Check sheet for the modelled part. Datum: model origin and axes. Units: mm. A direction names the side the tool comes from. Give positions to 0.01 mm unless a question says otherwise; leave off trailing zeros. Write each loop counter-clockwise with the first axis right and the second up, starting at its lowest first coordinate (ties: lowest second). Pieces come first, ordered by that corner, then holes. Notation, with made-up numbers: (26.5, 50) -> (73.5, 50) arc R31 ccw to (73.5, 81) -> close; hole circle Ø4 at (47.5, 87). An arc over 180 degrees is marked (long way). Use a Markdown table: item, result. Add a question column.
1. Set-up check for faces 4 (the flat face through (1.28, 21.51, 2.26)), 5 (the cylindrical face through (-3.417, 21.372, -0.759)): record each of +Z, -Z, +X, -X, +Y, -Y from which the full face is reachable in a straight line by a thin tool's end or side.
2. Release check for a two-part mould opening along Z. For faces 1 (the cylindrical face through (0.676, 9.86, 2.146)), 2 (the flat face through (3, 22, -1)), 3 (the flat face through (0, 21.016, 0)) record: released by +Z, released by -Z, zero draft, split by the parting line, or undercut.
3. Cross-section at B-B (y = 15.75). Enter the section's corners in (x, z), then the cut area to 3 significant figures.
4. Gauge pin test, flat ends, axial feed: P1, Ø1.5, axis at x = 0, y = 17, coming from the -Z side; P2, Ø1.6, axis at x = -1, z = 1, coming from the +Y side; P3, Ø2, axis at y = 3, z = 1, coming from the +X side. Record the tip position at first contact, or that the pin passes through.
5. Cross-section at A-A (z = 0). Enter the section's corners in (x, y), then the cut area to 3 significant figures.
6. Scan lines: probe 1 along Y at (x, z) = (-0.5, 0); probe 2 along Y at (x, z) = (1, 2.25); probe 3 along X at (y, z) = (20.75, -2). Record each from-to range of solid material in increasing order. Write a range as [from, to].
from build123d import *

# Parameters (mm, degrees)
SKETCH1_R      = 2.25
LENGTH_DEPTH   = 20
SKETCH2_R      = 3.5
CAP_DEPTH      = 2
CHAMFER_2_SIZE = 0.762
HEX_2_DEPTH    = 0.984


with BuildPart() as part:
    # Sketch1 → Length (new body)
    with BuildSketch(Plane(origin=(0, 0, 0), x_dir=(1, 0, 0), z_dir=(0, 1, 0))):
        with Locations(Location((0, 0, 0), (0, 0, 270))):
            Circle(SKETCH1_R)
    extrude(amount=LENGTH_DEPTH)

    # Sketch2 → Cap (add)
    with BuildSketch(Plane(origin=(0, 20, 0), x_dir=(1, 0, 0), z_dir=(0, 1, 0))):
        with Locations(Location((0, 0, 0), (0, 0, 270))):
            Circle(SKETCH2_R)
    extrude(amount=CAP_DEPTH)

    # Chamfer 2
    chamfer_2_edges = [part.edges().sort_by_distance(p)[0] for p in [
        (0, 20, -3.5),
    ]]
    chamfer(chamfer_2_edges, length=CHAMFER_2_SIZE)

    # Sketch3 → Hex 2 (cut)
    with BuildSketch(Plane(origin=(0, 22, 0), x_dir=(1, 0, 0), z_dir=(0, 1, 0))):
        Polygon((0, 3), (-2.598076211, 1.5), (-2.598076211, -1.5), (0, -3), (2.598076211, -1.5), (2.598076211, 1.5), align=None)
    extrude(amount=-HEX_2_DEPTH, mode=Mode.SUBTRACT)


solid = part.part
Worked answers:
| question | item | result |
|---|---|---|
| 1 | face 4 | +Y |
| 1 | face 5 | +Y, -Y |
| 2 | face 1 | split by the parting line |
| 2 | face 2 | zero draft |
| 2 | face 3 | undercut |
| 3 | outline | circle Ø4.5 at (0, 0) |
| 3 | area | 15.9 mm² |
| 4 | P1 | stops at z = -2.25 |
| 4 | P2 | stops at y = 21.02 |
| 4 | P3 | stops at x = 2.25 |
| 5 | outline | (-3.5, 20.76) -> (-2.74, 20) -> (-2.25, 20) -> (-2.25, 0) -> (2.25, 0) -> (2.25, 20) -> (2.74, 20) -> (3.5, 20.76) -> (3.5, 22) -> (2.6, 22) -> (2.6, 21.02) -> (-2.6, 21.02) -> (-2.6, 22) -> (-3.5, 22) -> close |
| 5 | area | 98.3 mm² |
| 6 | probe 1 | y = [0, 21.02] |
| 6 | probe 2 | y = [20, 21.02] |
| 6 | probe 3 | x = [-2.86, 2.86] |
